Input: part model. Units: mm. Frame: model coordinates. Face numbers are marked on the shaded views. Coordinates: 2 decimals unless noted, no trailing zeros. Write each loop counter-clockwise with the first axis right and the second up, starting at its lowest first coordinate (ties: lowest second). Pieces come first, ordered by that corner, then holes.
1) Section query B-B (y = 855). Output: boundary loops of the cut face in (x, z).
2) Line query: L1, parallel to Y at x = -52.75, z = 0; L2, parallel to Z at x = -1, y = 258.5; L3, parallel to X at y = 450, z = 0. Output: solid intervals per line, ascending.
3) Pin query (flat end, axial travel): pin 1 Ø12 at (x, y) = (-34, 697) entering from -Z; pin 2 Ø3 at (y, z) = (800.1, 0) entering from -X; pin 3 Ø5 at (y, z) = (359.5, -4.5) entering from +X; pin 4 Ø3 at (x, y) = (6, 333.5) entering from -Z. Return the tip coordinate at first contact, or that it passes through.
4) Section query A-A (z = 13.5). Output: boundary loops of the cut face in (x, y), then the cut area to 3 significant figures.
5) Draft query along X for the marked faces 1 and 2. Return one class per face: pulls with the +X half, pulls with the -X half, needs draft (parallel to the pull), parting line crosses it, or undercut.
from build123d import *

# Parameters (mm, degrees)
SKETCH1_R                 = 53.721
SKETCH1_R_2               = 50.8
BODY_TUBE_EXTRUSION_DEPTH = 1104.9
BULKHEAD_HOLE_REACH       = 1113.411
BULKHEAD_HOLE_END_RADIUS  = 50.8
SKETCH2_R                 = 1.6383
CIRPATTERN1_COUNT         = 8


with BuildPart() as part:
    # Sketch1 → Body Tube Extrusion (new body)
    with BuildSketch(Plane(origin=(0, 0, 0), x_dir=(1, 0, 0), z_dir=(0, 1, 0))):
        Circle(SKETCH1_R)
        Circle(SKETCH1_R_2, mode=Mode.SUBTRACT)
    extrude(amount=BODY_TUBE_EXTRUSION_DEPTH)

    # Bulkhead Hole: up to this cylinder (the profile starts outside it)
    bulkhead_hole_end = Plane(origin=(0, 800.1, 0), z_dir=(0, -1, 0)) * Cylinder(BULKHEAD_HOLE_END_RADIUS, 2329.422, mode=Mode.PRIVATE)
    # Sketch2 → Bulkhead Hole (cut, up to the surface)
    with BuildSketch(Plane.XY.offset(53.721), mode=Mode.PRIVATE) as bulkhead_hole_sk1:
        with Locations((0, 800.1)):
            Circle(SKETCH2_R)
    bulkhead_hole_tool1 = extrude(bulkhead_hole_sk1.sketch, amount=-BULKHEAD_HOLE_REACH, mode=Mode.PRIVATE) - bulkhead_hole_end
    bulkhead_hole = bulkhead_hole_tool1.solids().sort_by_distance((0, 800.1, 53.721))[0]
    add(bulkhead_hole, mode=Mode.SUBTRACT)

    # CirPattern1: Bulkhead Hole ×8 about axis
    cirpattern1_axis = Axis((0, 1104.9, 0), (0, -1, 0))
    for i in range(1, CIRPATTERN1_COUNT):
        add(bulkhead_hole.rotate(cirpattern1_axis, i * 360 / CIRPATTERN1_COUNT), mode=Mode.SUBTRACT)


solid = part.part
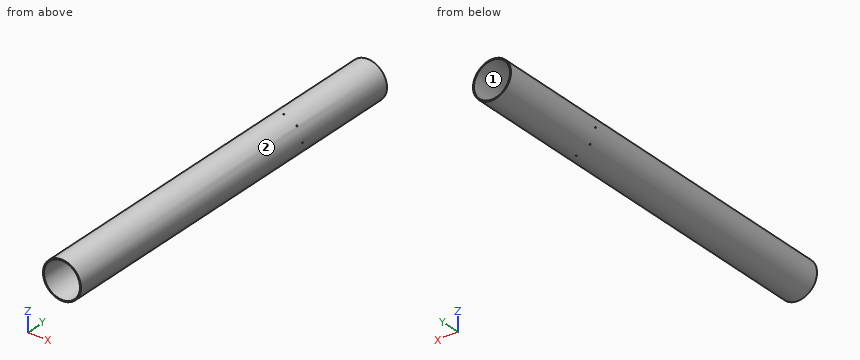
Answer:
1. outline: circle Ø107.44 at (0, 0); hole circle Ø101.6 at (0, 0)
2. L1: y = 0 to 798.46, 801.74 to 1104.9
2. L2: z = -53.71 to -50.79, 50.79 to 53.71
2. L3: x = -53.72 to -50.8, 50.8 to 53.72
3. pin 1: stops at z = -45.85
3. pin 2: passes through
3. pin 3: stops at x = 53.68
3. pin 4: stops at z = -53.53
4. outline: (-52, 0) - (-48.97, 0) - (-48.97, 1104.9) - (-52, 1104.9) - close; (48.97, 0) - (52, 0) - (52, 1104.9) - (48.97, 1104.9) - close
4. area: 6,680 mm2
5. face 1: undercut
5. face 2: parting line crosses it
